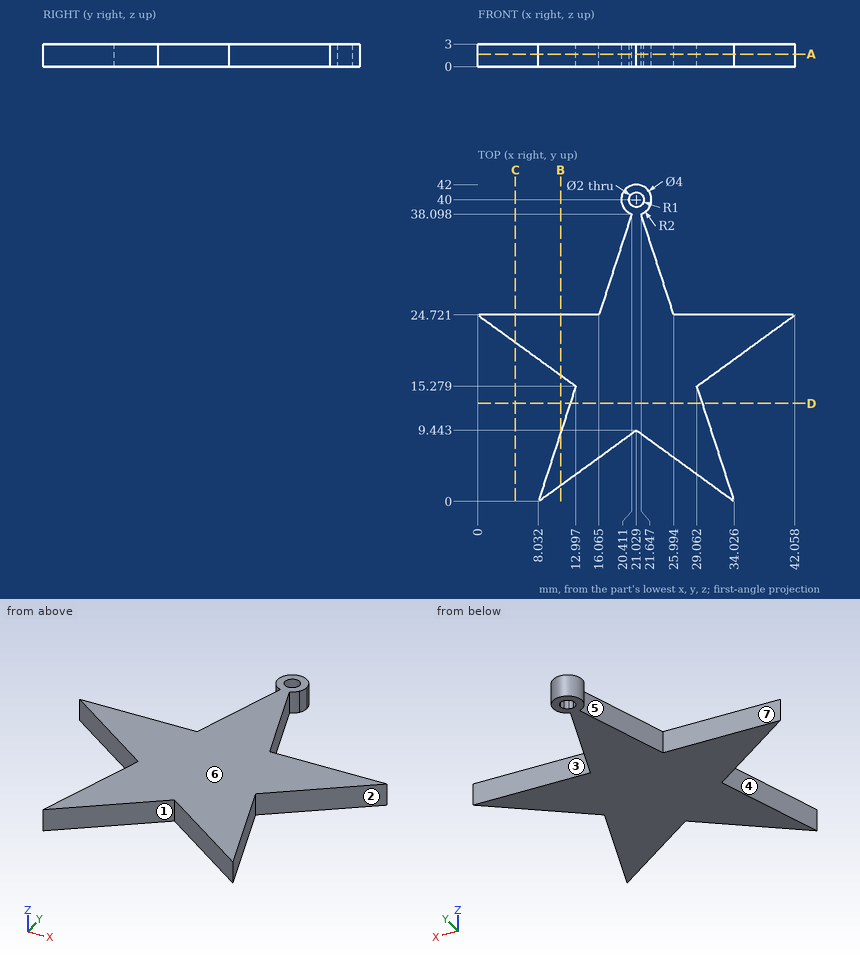
Here's the drawing with two shaded views (mm, measured from the low corner). I have some questions. A direction names the side the tool comes from. Give positions to 0.01 mm unless a question says otherwise; leave off trailing zeros. Loops run counter-clockwise (first coordinate to the right, second up) from the corner with the lowest first, then second, coordinate; pieces in that order, holes last. Notation, with made-up numbers: M 61,7 L 80,7 A28 ccw 80,42 Z; hole C 4.25,-13.75 d7. An arc over 180 degrees is marked long. Use one line per item in the form item = value. Start each with the question number.
(1) I want a section at B-B, the plane x = 11. Write out the boundary of the cut face in (y, z), and give its area (3 significant figures).
(2) I want a section at A-A, the plane z = 1.65. Write out the boundary of the cut face in (x, y) (1 decimal), and give its area (3 significant figures).
(3) I want a section at C-C, the plane x = 5. Write out the boundary of the cut face in (y, z), and give its area (3 significant figures).
(4) Thinking about a two-plate mould opening in X: for the marked faces 1, 2, 3 and 4, which applies, released by +X, released by -X, zero draft, split by the parting line, or undercut?
(5) I'm going to push flat-ended pins straight in: P1, Ø1.8, axis at x = 21.03, y = 40, coming from the +Z side (3 decimals); P2, Ø0.9, axis at x = 37, z = 1, coming from the +Y side. Where does each tip first touch, or does it pass through?
(6) Please list where these lines run through material, in increasing order: line 1 (X direction, y = 40, z = 1.95); line 2 (Y direction, x = 20.5, z = 1.45); line 3 (X direction, y = 8.5, z = 0.3) (1 decimal).
(7) I want a section at D-D, the plane y = 13. Write out the boundary of the cut face in (x, z).
(8) On a 3-axis mill with a long thin cutter (end or side, diameter ignored), from which of +Z, -Z, +X, -X, +Y, -Y can I reach the whole of each face in a straight line? I mean the marked faces 5, 6 and 7. Say none if no direction works.
Worked out:
q1.outline = M 2.16,0 L 9.13,0 L 9.13,3 L 2.16,3 Z; M 16.73,0 L 24.72,0 L 24.72,3 L 16.73,3 Z
q1.area = 44.9 mm²
q2.outline = M 0,24.7 L 13,15.3 L 8,0 L 21,9.4 L 34,0 L 29.1,15.3 L 42.1,24.7 L 26,24.7 L 21.6,38.1 A2 ccw long 20.4,38.1 L 16.1,24.7 Z; hole C 21,40 d2
q2.area = 557 mm²
q3.outline = M 21.09,0 L 24.72,0 L 24.72,3 L 21.09,3 Z
q3.area = 10.9 mm²
q4.face_1 = undercut
q4.face_2 = released by +X
q4.face_3 = zero draft
q4.face_4 = released by -X
q5.P1 = through
q5.P2 = 24.72
q6.line_1 = 19.03 to 20.03, 22.03 to 23.03
q6.line_2 = 9.06 to 39.15, 40.85 to 41.93
q6.line_3 = 10.8 to 19.7, 22.3 to 31.3
q7.outline = M 12.26,0 L 29.8,0 L 29.8,3 L 12.26,3 Z
q8.face_5 = +Z, -Z, -X
q8.face_6 = +Z, +X, -X, +Y, -Y
q8.face_7 = +Z, -Z, -X, +Y
